```python
from build123d import *

# Parameters (mm, degrees)
SKETCH1_W               = 254
SKETCH1_H               = 88.9
SKETCH1_R               = 9.5
SKETCH1_W_2             = 27
SKETCH1_H_2             = 55
BOSS_EXTRUDE1_DEPTH     = 6.35
SKETCH4_W               = 19.05
SKETCH4_H               = 19.05
BOSS_EXTRUDE2_DEPTH     = 6.35
SKETCH7_W               = 34.925
SKETCH7_H               = 88.9
SKETCH7_W_2             = 50.8
BOSS_EXTRUDE3_DEPTH     = 6.35
F_1_4_CLEARANCE_HOLE1_D = 6.7564
FILLET1_R               = 3.175
FILLET2_R               = 7.62
CUT_EXTRUDE1_DEPTH      = 7.35


with BuildPart() as part:
    # Sketch1 → Boss-Extrude1 (new body)
    with BuildSketch(Plane(origin=(0, 0, 0), x_dir=(-1, 0, 0), z_dir=(0, 0, -1))):
        Rectangle(SKETCH1_W, SKETCH1_H)
        with Locations((-88.9000016, 14)):
            Circle(SKETCH1_R, mode=Mode.SUBTRACT)
        with Locations((-88.9000016, -14)):
            Circle(SKETCH1_R, mode=Mode.SUBTRACT)
        Rectangle(SKETCH1_W_2, SKETCH1_H_2, mode=Mode.SUBTRACT)
    extrude(amount=-BOSS_EXTRUDE1_DEPTH)

    # Sketch4 → Boss-Extrude2 (add)
    with BuildSketch(Plane.XY.offset(6.35)):
        with Locations((-107.95, 53.975)):
            Rectangle(SKETCH4_W, SKETCH4_H)
        with Locations((-107.95, -53.975)):
            Rectangle(SKETCH4_W, SKETCH4_H)
        with Locations((95.25, -53.975)):
            Rectangle(SKETCH4_W, SKETCH4_H)
        with Locations((95.25, 53.975)):
            Rectangle(SKETCH4_W, SKETCH4_H)
    extrude(amount=-BOSS_EXTRUDE2_DEPTH)

    # Sketch7 → Boss-Extrude3 (add)
    with BuildSketch(Plane.XY.offset(6.35)):
        with Locations((-144.4625, 0)):
            Rectangle(SKETCH7_W, SKETCH7_H)
        with Locations((152.4, 0)):
            Rectangle(SKETCH7_W_2, SKETCH7_H)
    extrude(amount=-BOSS_EXTRUDE3_DEPTH)

    # 1/4 Clearance Hole1 (through all)
    with Locations(Plane.XY.offset(6.35)):
        with Locations((-107.95, 53.975), (95.25, 53.975), (95.25, -53.975), (-107.95, -53.975), (168.275, -34.925), (168.275, 34.925), (-152.4, 34.925), (-152.4, -34.925), (-34.675, 17.4625), (-34.675, -17.4625)):
            Hole(F_1_4_CLEARANCE_HOLE1_D / 2)

    # Fillet1
    fillet1_edges = [part.edges().sort_by_distance(p)[0] for p in [
        (13.5, 27.5, 3.175),
        (-13.5, 27.5, 3.175),
        (-13.5, -27.5, 3.175),
        (13.5, -27.5, 3.175),
    ]]
    fillet(fillet1_edges, radius=FILLET1_R)

    # Fillet2
    fillet2_edges = [part.edges().sort_by_distance(p)[0] for p in [
        (-98.425, 44.45, 3.175),
        (-98.425, 63.5, 3.175),
        (-117.475, 63.5, 3.175),
        (-117.475, 44.45, 3.175),
        (-98.425, -63.5, 3.175),
        (-98.425, -44.45, 3.175),
        (-117.475, -44.45, 3.175),
        (-117.475, -63.5, 3.175),
        (85.725, -63.5, 3.175),
        (104.775, -63.5, 3.175),
        (104.775, -44.45, 3.175),
        (85.725, -44.45, 3.175),
        (85.725, 63.5, 3.175),
        (85.725, 44.45, 3.175),
        (104.775, 44.45, 3.175),
        (104.775, 63.5, 3.175),
        (-161.925, 44.45, 3.175),
        (-161.925, -44.45, 3.175),
        (177.8, -44.45, 3.175),
        (177.8, 44.45, 3.175),
    ]]
    fillet(fillet2_edges, radius=FILLET2_R)

    # Sketch8 → Cut-Extrude1 (cut, through all)
    with BuildSketch(Plane(origin=(0, 0, 0), x_dir=(-1, 0, 0), z_dir=(0, 0, -1))):
        with BuildLine():
            Line((10.325, 30.675), (-10.325, 30.675))
            ThreePointArc((-10.325, 30.675), (-14.815128061, 28.815128061), (-16.675, 24.325))
            Line((-16.675, 24.325), (-16.675, -24.325))
            ThreePointArc((-16.675, -24.325), (-14.815128061, -28.815128061), (-10.325, -30.675))
            Line((-10.325, -30.675), (10.325, -30.675))
            ThreePointArc((10.325, -30.675), (14.815128061, -28.815128061), (16.675, -24.325))
            Line((16.675, -24.325), (16.675, 24.325))
            ThreePointArc((16.675, 24.325), (14.815128061, 28.815128061), (10.325, 30.675))
        make_face()
        with BuildLine():
            Line((10.325, 27.5), (-10.325, 27.5))
            ThreePointArc((-10.325, 27.5), (-12.57006403, 26.57006403), (-13.5, 24.325))
            Line((-13.5, 24.325), (-13.5, -24.325))
            ThreePointArc((-13.5, -24.325), (-12.57006403, -26.57006403), (-10.325, -27.5))
            Line((-10.325, -27.5), (10.325, -27.5))
            ThreePointArc((10.325, -27.5), (12.57006403, -26.57006403), (13.5, -24.325))
            Line((13.5, -24.325), (13.5, 24.325))
            ThreePointArc((13.5, 24.325), (12.57006403, 26.57006403), (10.325, 27.5))
        make_face(mode=Mode.SUBTRACT)
    extrude(amount=-CUT_EXTRUDE1_DEPTH, mode=Mode.SUBTRACT)


solid = part.part
```
Source: CAD feature listing. Evaluate the final solid. Frame: model axes, mm. A direction names the side the tool comes from. Give positions to 0.01 mm unless a question says otherwise; leave off trailing zeros. Loops run counter-clockwise (first coordinate to the right, second up) from the corner with the lowest first, then second, coordinate; pieces in that order, holes last. Notation, with made-up numbers: (-10.5, 71) - (8.5, 71) arc R13 cw to (8.5, 90) - close; hole circle Ø1 at (-30.75, 12). An arc over 180 degrees is marked (long way). Use CSV: the item, a comma, the result in double quotes.
1) Pin query (flat end, axial travel): P1, Ø1.1, axis at y = 54.5, z = 2.5, coming from the -X side (3 decimals); P2, Ø1.9, axis at y = 54.5, z = 2, coming from the +X side (3 decimals). Return the tip coordinate at first contact, or that it passes through.
Worked out:
P1,"stops at x = -117.475"
P2,"stops at x = 104.775"
2) Cut plane B-B (z = 3). Count the separate pieces of the cut face and the enclosed holes in it, and give its area (3 significant figures).
Worked out:
separate pieces,"1"
enclosed holes,"13"
area,"28,700 mm^2"
3) Set-up query: faces 1 (the cylindrical face through (175.509, 42.277, 3.131)), 2 (the cylindrical face through (-119.77, -46.62, 3.13)), 3 (the cylindrical face through (-96.25, -46.74, 3.13)), 4 (the flat face through (-140, 44.45, 3)), 5 (the cylindrical face through (14.77, 28.86, 3.13)). Return all of +Z, -Z, +X, -X, +Y, -Y with unobstructed straight access to the full face (end or side cutting, diameter ignored); none if empty.
Worked out:
face 1,"+Z, -Z, +X, +Y"
face 2,"+Z, -Z, -X, -Y"
face 3,"+Z, -Z, -Y"
face 4,"+Z, -Z, -X, +Y"
face 5,"+Z, -Z"
4) Line query: line 1 (Y direction, x = -152.4, z = 4.75); line 2 (X direction, y = 13.5, z = 4.75) (3 decimals); line 3 (X direction, y = 54.5, z = 2.75) (3 decimals). Output: solid intervals per line, ascending.
Worked out:
line 1,"y = -44.45 to -38.3, -31.55 to 31.55, 38.3 to 44.45"
line 2,"x = -161.925 to -16.675, 16.675 to 79.413, 98.387 to 177.8"
line 3,"x = -117.475 to -111.287, -104.613 to -98.425, 85.725 to 91.913, 98.587 to 104.775"
5) Mould query, pull axis Y, two halves, no side actions, for faces 6 (the flat face through (-140, -44.45, 3)), 7 (the cylindrical face through (92.13, 52.68, 3.13)), 8 (the cylindrical face through (-100.72, 61.33, 3.13)). Classes: +Y half, -Y half, draft (parallel to the pull), parting line (faces both ways), or undercut.
Worked out:
face 6,"-Y half"
face 7,"undercut"
face 8,"+Y half"
6) Cut plane A-A (x = -25). Output: boundary loops of the cut face in (y, z), and give its area (3 significant figures).
Worked out:
outline,"(-44.45, 0) - (44.45, 0) - (44.45, 6.35) - (-44.45, 6.35) - close"
area,"565 mm^2"
